Autodesk Inventor part; units mm, degrees
ref_plane "YZ Plane" through (0, 0, 0) normal (1, 0, 0) x (0, 1, 0)
ref_plane "XZ Plane" through (0, 0, 0) normal (0, 1, 0) x (-1, 0, 0)
ref_plane "XY Plane" through (0, 0, 0) normal (0, 0, 1) x (1, 0, 0)
sketch "Esquisse1" plane through (0, 0, 0) normal (0, 1, 0) x (-1, 0, 0)
  circle A0 centre (0, 0) radius 5.3
  dimension "d0" = 10.6
extrude "Extrusion1" add sketch "Esquisse1" along normal blind 7
shell "Coque2" thickness 1.7 removed faces 1 at (-1.6995, 0, -1.9343)
sketch "Esquisse6" plane through (0, 5.3, 0) normal (0, -1, 0) x (1, 0, 0)
  circle A0 centre (0, 0) radius 2.5
  circle A1 centre (0, 0) radius 1.5
  dimension "d20" = 5
  dimension "d21" = 3
extrude "Extrusion4" add sketch "Esquisse6" along normal blind 4
sketch "Esquisse7" plane through (0, 0, 0) normal (0, -1, 0) x (1, 0, 0)
  line L0 (-8, 1) -> (-4.8, 1)
  line L1 (-4.8, 1) -> (-4.8, -1)
  line L2 (-4.8, -1) -> (-8, -1)
  line L3 (-8, -1) -> (-8, 1)
  line L4 (4.8, 1) -> (8, 1)
  line L5 (8, 1) -> (8, -1)
  line L6 (8, -1) -> (4.8, -1)
  line L7 (4.8, -1) -> (4.8, 1)
  point P0 (0, 0)
  dimension "d24" = 2
  dimension "d25" = 1
  dimension "d26" = 4.8
  dimension "d27" = 4.8
  dimension "d29" = 8
  dimension "d30" = 8
extrude "Extrusion5" add sketch "Esquisse7" against normal blind 2
fillet "Congé3" radius 0.1 1 edges at (5.3, 7, 0)
chamfer "Chanfrein1" distance 0.3 angle 45 1 edges at (3.6, 0, 0)
properties part number "Button-SNES" material "Plastique ABS"
Here's how the part is built. I have some questions about the finished solid (model axes, mm). A direction names the side the tool comes from. Coordinates: 2 decimals unless noted, no trailing zeros. Loops run counter-clockwise (first coordinate to the right, second up) from the corner with the lowest first, then second, coordinate; pieces in that order, holes last. Notation, with made-up numbers: (45, -28) -> (81, -28) arc R17 ccw to (81, -4) -> close; hole circle Ø7 at (72.25, 33). An arc over 180 degrees is marked (long way). Use one line per item in the form item = value. Start each with the question number.
(1) Please list where these lines run through material, in increasing order: line 1 along Z through (x, y) = (0, 2.4); line 2 along Z through (x, y) = (-2.25, 2.75); line 3 along X through (y, z) = (3.25, 0.5).
(2) If we section it at B-B (z = 0): Please give me the cut outline in (x, y), then the cut area to 3 significant figures.
(3) If we section it at D-D (y = 5.5): Please give me the cut outline in (x, z), then the cut area to 3 significant figures.
(4) If we section it at C-C (x = 0): Please give me the cut outline in (y, z).
(5) If we section it at A-A (y = 2.5): Please give me the cut outline in (x, z).
(6) Will these pins go through, and if not, where does the flat tip stop? pin 1 (0.6 mm diameter, centred on x = 6, z = 0, fed in from +Y); pin 2 (4 mm diameter, centred on y = 2, z = -4, fed in from -X); pin 3 (2 mm diameter, centred on x = 7, y = 1, fed in from +Z).
(7) We'd pull the mould along X, two halves only. Please class faces 6 (the face through (-0.54, 3.33, 2.44)), 7 (the face through (-4.896, 3.402, 2.03)), 8 (the face through (4, 0, -2)), 9 (the face through (0.9, 5.3, 2.5)): pulls with the +X half, pulls with the -X half, needs draft (parallel to the pull), parting line crosses it, or undercut.
(8) On a 3-axis mill with a long thin cutter (end or side, diameter ignored), from which of +Z, -Z, +X, -X, +Y, -Y can I reach the whole of each face in a straight line? I mean faces 1 (the face through (7, 1, -1)), 2 (the face through (-7, 1, -1)), 3 (the face through (7, 1, 1)), 4 (the face through (-7, 1, 1)), 5 (the face through (-1.5, 3.33, -0.07)). Say none if no direction works.
Verdict:
q1.line_1 = -5.3 to -3.6, -2.5 to -1.5, 1.5 to 2.5, 3.6 to 5.3
q1.line_2 = -4.8 to -2.81, -1.09 to 1.09, 2.81 to 4.8
q1.line_3 = -5.28 to -3.57, -2.45 to -1.41, 1.41 to 2.45, 3.57 to 5.28
q2.outline = (-8, 0) -> (-3.9, 0) -> (-3.6, 0.3) -> (-3.6, 5.3) -> (-2.5, 5.3) -> (-2.5, 1.3) -> (-1.5, 1.3) -> (-1.5, 5.3) -> (1.5, 5.3) -> (1.5, 1.3) -> (2.5, 1.3) -> (2.5, 5.3) -> (3.6, 5.3) -> (3.6, 0.3) -> (3.9, 0) -> (8, 0) -> (8, 2) -> (5.3, 2) -> (5.3, 6.9) arc R0.1 ccw to (5.2, 7) -> (-5.2, 7) arc R0.1 ccw to (-5.3, 6.9) -> (-5.3, 2) -> (-8, 2) -> close
q2.area = 54.7 mm²
q3.outline = circle Ø10.6 at (0, 0)
q3.area = 88.2 mm²
q4.outline = (0, -5.3) -> (6.9, -5.3) arc R0.1 ccw to (7, -5.2) -> (7, 5.2) arc R0.1 ccw to (6.9, 5.3) -> (0, 5.3) -> (0, 3.9) -> (0.3, 3.6) -> (5.3, 3.6) -> (5.3, 2.5) -> (1.3, 2.5) -> (1.3, 1.5) -> (5.3, 1.5) -> (5.3, -1.5) -> (1.3, -1.5) -> (1.3, -2.5) -> (5.3, -2.5) -> (5.3, -3.6) -> (0.3, -3.6) -> (0, -3.9) -> close
q5.outline = circle Ø10.6 at (0, 0); circle Ø5 at (0, 0); hole circle Ø7.2 at (0, 0); hole circle Ø3 at (0, 0)
q6.pin_1 = 2
q6.pin_2 = -4.91
q6.pin_3 = 1
q7.face_6 = undercut
q7.face_7 = parting line crosses it
q7.face_8 = needs draft
q7.face_9 = undercut
q8.face_1 = -Z, +X, +Y, -Y
q8.face_2 = -Z, -X, +Y, -Y
q8.face_3 = +Z, +X, +Y, -Y
q8.face_4 = +Z, -X, +Y, -Y
q8.face_5 = -Y
